```python
from build123d import *
from build123d import SkipClean  # not in build123d's __all__

# Parameters (mm, degrees)
F1_DEPTH      = 21
F2_DEPTH      = 3
F0_R          = 19.05
F0_R_2        = 5.715
F3_DEPTH      = 1.6
F3_DEPTH_BACK = 10
F0_W          = 56.134
F0_H          = 56.134
F0_R_3        = 2.55
F4_DEPTH      = 4.9022
F6_DEPTH      = 75.819
F7_R          = 2
F8_W          = 11.938
F8_H          = 11.938
F9_DEPTH      = 1


with BuildPart() as f1:
    # F0 (on Front) → F1 (new body)
    with BuildSketch(Plane.XZ):
        with BuildLine():
            ThreePointArc((-1.7102631376, 2.675), (-1.5248835264, -2.7848438432), (3.175, 0))
            ThreePointArc((3.175, 0), (2.7848438432, 1.5248835264), (1.7102631376, 2.675))
            Line((1.7102631376, 2.675), (-1.7102631376, 2.675))
        make_face()
    extrude(amount=F1_DEPTH)

    # F0 (on Front) → F2 (join, symmetric)
    with BuildSketch(Plane.XZ):
        with BuildLine():
            Line((-1.7102631376, 2.675), (1.7102631376, 2.675))
            ThreePointArc((1.7102631376, 2.675), (0, 3.175), (-1.7102631376, 2.675))
        make_face()
        with BuildLine():
            ThreePointArc((-1.7102631376, 2.675), (-1.5248835264, -2.7848438432), (3.175, 0))
            ThreePointArc((3.175, 0), (2.7848438432, 1.5248835264), (1.7102631376, 2.675))
            Line((1.7102631376, 2.675), (-1.7102631376, 2.675))
        make_face()
    with SkipClean():  # cleaning this boolean's faces spoils the solid; the shape is the same uncleaned
        extrude(amount=F2_DEPTH, both=True)



with BuildPart() as f3:
    # F0 (on Front) → F3 (new body, two sides)
    with BuildSketch(Plane.XZ) as f3_sk:
        Circle(F0_R)
        Circle(F0_R_2, mode=Mode.SUBTRACT)
    extrude(amount=F3_DEPTH)
    extrude(f3_sk.sketch, amount=-F3_DEPTH_BACK)

    # F0 (on Front) → F4 (join)
    with BuildSketch(Plane.XZ):
        Rectangle(F0_W, F0_H)
        with Locations((-23.5, -23.5)):
            Circle(F0_R_3, mode=Mode.SUBTRACT)
        with Locations((23.5, -23.5)):
            Circle(F0_R_3, mode=Mode.SUBTRACT)
        with Locations((-23.5, 23.5)):
            Circle(F0_R_3, mode=Mode.SUBTRACT)
        Circle(F0_R, mode=Mode.SUBTRACT)
        with Locations((23.5, 23.5)):
            Circle(F0_R_3, mode=Mode.SUBTRACT)
    extrude(amount=-F4_DEPTH)


with BuildPart() as f1_1:
    add(f1.part, clean=False)

    with SkipClean():  # cleaning this boolean's faces spoils the solid; the shape is the same uncleaned
        add(f3.part)  # F6 merges F3
    # F5 (on Front) → F6 (join)
    with BuildSketch(Plane.XZ):
        with BuildLine():
            ThreePointArc((-19.05, 23.5), (-20.3533748237, 20.3533748237), (-23.5, 19.05))
            Line((-23.5, 19.05), (-28.067, 19.05))
            Line((-28.067, 19.05), (-28.067, -19.05))
            Line((-28.067, -19.05), (-23.5, -19.05))
            ThreePointArc((-23.5, -19.05), (-20.3533748237, -20.3533748237), (-19.05, -23.5))
            Line((-19.05, -23.5), (-19.05, -28.067))
            Line((-19.05, -28.067), (19.05, -28.067))
            Line((19.05, -28.067), (19.05, -23.5))
            ThreePointArc((19.05, -23.5), (20.3533748237, -20.3533748237), (23.5, -19.05))
            Line((23.5, -19.05), (28.067, -19.05))
            Line((28.067, -19.05), (28.067, 19.05))
            Line((28.067, 19.05), (23.5, 19.05))
            ThreePointArc((23.5, 19.05), (20.3533748237, 20.3533748237), (19.05, 23.5))
            Line((19.05, 23.5), (19.05, 28.067))
            Line((19.05, 28.067), (-19.05, 28.067))
            Line((-19.05, 28.067), (-19.05, 23.5))
        make_face()
    with SkipClean():  # cleaning this boolean's faces spoils the solid; the shape is the same uncleaned
        extrude(amount=-F6_DEPTH)

    # F7
    f7_edges = [f1_1.edges().sort_by_distance(p)[0] for p in [
        (19.05, 40.3606, 28.067),
        (28.067, 40.3606, 19.05),
        (28.067, 2.4511, 28.067),
        (28.067, 2.4511, -28.067),
        (28.067, 40.3606, -19.05),
        (19.05, 40.3606, -28.067),
        (-19.05, 40.3606, -28.067),
        (-28.067, 40.3606, -19.05),
        (-28.067, 2.4511, -28.067),
        (-28.067, 2.4511, 28.067),
        (-28.067, 40.3606, 19.05),
        (-19.05, 40.3606, 28.067),
    ]]
    fillet(f7_edges, radius=F7_R)

    # F8 (on face) → F9 (join)
    with BuildSketch(Plane.YZ.offset(28.067)):
        with Locations((69.85, 0)):
            Rectangle(F8_W, F8_H)
    extrude(amount=F9_DEPTH)


solid = f1_1.part
```
Check sheet for the modelled part. Datum: model origin and axes. Units: mm. A direction names the side the tool comes from. Coordinates: 2 decimals unless noted, no trailing zeros. Order: outer loops, then holes, each group sorted by start corner. A loop starts at its lowest first (then second) coordinate and runs counter-clockwise, first axis right, second up. Notation, with made-up numbers: M 9,0.5 L 46,0.5 A10 cw 46,19.5 Z; hole C -19.5,49.25 d8. An arc over 180 degrees is marked long. One line per question, with ' | ' between items. Start each with the question number.
Item 1: Material ranges on line 1 (Z direction, x = 23.5, y = 2.7); line 2 (Y direction, x = -3.5, z = 7.5); line 3 (X direction, y = 66.5, z = 17), recorded low to high.
Item 2: Sectioned sample at B-B on x = 0. Record the cut outline in (y, z) (3 decimals).
Item 3: Gauge pin test, flat ends, axial feed: P1, Ø1.3, axis at y = 33.5, z = -25.5, coming from the +X side; P2, Ø3, axis at x = -25, y = 48.5, coming from the +Z side; P3, Ø3.5, axis at x = 25, z = -25, coming from the +Y side; P4, Ø3, axis at x = -23.5, z = -23.5, coming from the +Y side. Record the tip position at first contact, or that the pin passes through.
Item 4: Sectioned sample at A-A on y = 37. Record the cut outline in (x, z).
Item 5: Sectioned sample at D-D on z = -11. Record the cut outline in (x, y).
Item 6: Mould release check, pull along Z, two halves, no side actions. Record for faces 1 (the flat face through (4, -1.6, 5)), 2 (the flat face through (-25, 40, -19.05)), 3 (the cylindrical face through (5.45, -0.79, 1.72)): pulls with the +Z half, pulls with the -Z half, needs draft (parallel to the pull), parting line crosses it, or undercut.
Item 7: Access from +Z, -Z, +X, -X, +Y, -Y to the whole of each face (thin tool, end or side, straight path). Record for faces 4 (the flat face through (25, 40, -19.05)), 5 (the flat face through (25, 40, 19.05)), 6 (the flat face through (-7, 0, 19)).
Item 8: Sectioned sample at C-C on z = 8.5. Record the cut outline in (x, y), and give its area (3 significant figures).
Answer below:
1) line 1: z = -28.07 to -26.05, -20.95 to 20.95, 26.05 to 28.07 | line 2: y = -1.6 to 75.82 | line 3: x = -28.07 to 28.07
2) outline: M -21,-3.175 L 0,-3.175 L 0,-5.715 L -1.6,-5.715 L -1.6,-19.05 L 0,-19.05 L 0,-28.067 L 75.819,-28.067 L 75.819,28.067 L 0,28.067 L 0,19.05 L -1.6,19.05 L -1.6,5.715 L 0,5.715 L 0,3.175 L -3,3.175 L -3,2.675 L -21,2.675 Z
3) P1: stops at x = 19.05 | P2: stops at z = 19.05 | P3: stops at y = 4.9 | P4: passes through
4) outline: M -28.07,-17.05 A2 ccw -26.07,-19.05 L -23.5,-19.05 A4.45 cw -19.05,-23.5 L -19.05,-26.07 A2 ccw -17.05,-28.07 L 17.05,-28.07 A2 ccw 19.05,-26.07 L 19.05,-23.5 A4.45 cw 23.5,-19.05 L 26.07,-19.05 A2 ccw 28.07,-17.05 L 28.07,17.05 A2 ccw 26.07,19.05 L 23.5,19.05 A4.45 cw 19.05,23.5 L 19.05,26.07 A2 ccw 17.05,28.07 L -17.05,28.07 A2 ccw -19.05,26.07 L -19.05,23.5 A4.45 cw -23.5,19.05 L -26.07,19.05 A2 ccw -28.07,17.05 Z
5) outline: M -28.07,0 L -15.55,0 L -15.55,-1.6 L 15.55,-1.6 L 15.55,0 L 28.07,0 L 28.07,75.82 L -28.07,75.82 Z
6) face 1: needs draft | face 2: pulls with the -Z half | face 3: undercut
7) face 4: -Z, +X, +Y | face 5: +Z, +X, +Y | face 6: -Y
8) outline: M -28.07,0 L -17.05,0 L -17.05,-1.6 L 17.05,-1.6 L 17.05,0 L 28.07,0 L 28.07,75.82 L -28.07,75.82 Z | area: 4,310 mm^2
